Geometry: final body of the model. Coordinates: model frame, mm. Face numbers are marked on the shaded views. A direction names the side the tool comes from. Coordinates: 2 decimals unless noted, no trailing zeros. Order: outer loops, then holes, each group sorted by start corner. A loop starts at its lowest first (then second) coordinate and runs counter-clockwise, first axis right, second up. Notation, with made-up numbers: (-31.75, -26) - (16.25, -26) arc R16 cw to (16.25, -8) - close; hole circle Ø6 at (43, 58). An arc over 180 degrees is marked (long way). Use a Markdown table: item, result. Add a question column.
```python
from build123d import *

# Parameters (mm, degrees)
F1_DEPTH       = 35
F3_D           = 5
F3_START       = 1.7550021
F3_CBORE_D     = 10
F3_CBORE_DEPTH = 8
F4_W           = 22.4
F4_H           = 2
F5_DEPTH       = 25
F6_R           = 6
F7_DEPTH       = 8


with BuildPart() as f1:
    # F0 (on Top) → F1 (new body, symmetric)
    with BuildSketch(Plane.XY):
        with BuildLine():
            ThreePointArc((-17.3192642082, 2.5086026559), (17.5, 0), (-17.3192642082, -2.5086026559))
            Line((-17.3192642082, -2.5086026559), (-20.3459311096, -2.5086026559))
            ThreePointArc((-20.3459311096, -2.5086026559), (-16.3392263155, -12.3806172468), (-7.9192642082, -18.9086026559))
            ThreePointArc((-7.9192642082, -18.9086026559), (20.5, 0), (-7.9192642082, 18.9086026559))
            Line((-7.9192642082, 18.9086026559), (-20.1192642082, 18.9086026559))
            ThreePointArc((-20.1192642082, 18.9086026559), (-25.7761184577, 16.5654569054), (-28.1192642082, 10.9086026559))
            Line((-28.1192642082, 10.9086026559), (-28.1192642082, 2.5086026559))
            Line((-28.1192642082, 2.5086026559), (-17.3192642082, 2.5086026559))
        make_face()
        with BuildLine():
            ThreePointArc((-7.9192642082, -18.9086026559), (-16.3392263155, -12.3806172468), (-20.3459311096, -2.5086026559))
            Line((-20.3459311096, -2.5086026559), (-28.1192642082, -2.5086026559))
            Line((-28.1192642082, -2.5086026559), (-28.1192642082, -10.9086026559))
            ThreePointArc((-28.1192642082, -10.9086026559), (-25.7761184577, -16.5654569054), (-20.1192642082, -18.9086026559))
            Line((-20.1192642082, -18.9086026559), (-7.9192642082, -18.9086026559))
        make_face()
    extrude(amount=F1_DEPTH, both=True)

    # F3 (through all)
    # its depths count from where the whole tool has entered the part; down to there all is cleared
    with Locations(Plane(origin=(0, 18.9086026559, 0), x_dir=(-1, 0, 0), z_dir=(0, 1, 0)).offset(-F3_START)):
        with Locations((20.1192642082, 24.25), (20.1192642082, 9.25), (20.1192642082, -9.25), (20.1192642082, -24.25)):
            CounterBoreHole(F3_D / 2, F3_CBORE_D / 2, F3_CBORE_DEPTH)

    # F4 (on Front) → F5 (cut, symmetric)
    with BuildSketch(Plane.XZ):
        with Locations((-16.9192642082, 0)):
            Rectangle(F4_W, F4_H)
    extrude(amount=F5_DEPTH, both=True, mode=Mode.SUBTRACT)

    # F6 (on face) → F7 (cut)
    with BuildSketch(Plane.XY.offset(35)):
        with Locations((0.8263058844, -25)):
            Circle(F6_R)
        with Locations((18.2619560239, -17.0933830355)):
            Circle(F6_R)
        with Locations((25, 0.8263058844)):
            Circle(F6_R)
        with Locations((17.0933830355, 18.2619560239)):
            Circle(F6_R)
        with Locations((-0.8263058844, 25)):
            Circle(F6_R)
    extrude(amount=-F7_DEPTH, mode=Mode.SUBTRACT)


solid = f1.part
```
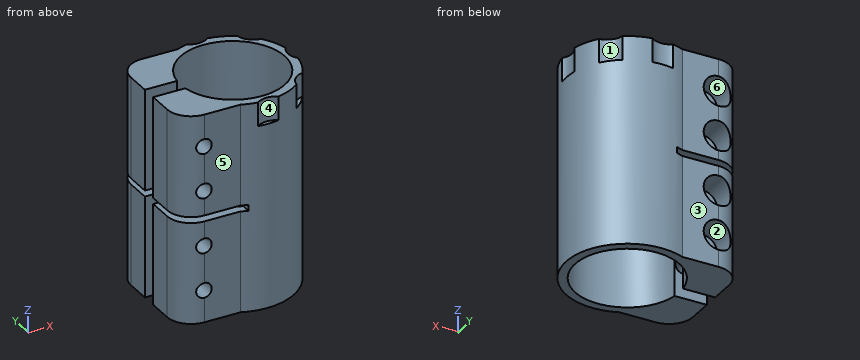
1) Set-up query: the marked faces 4, 5 and 6. Return all of +Z, -Z, +X, -X, +Y, -Y with unobstructed straight access to the full face (end or side cutting, diameter ignored); none if empty.
2) Pin query (flat end, axial travel): pin 1 (0.7 mm diameter, centred on x = -0.5, y = 19.5, fed in from +Z); pin 2 (8 mm diameter, centred on x = -20.12, z = 24.25, fed in from -Y); pin 3 (3.5 mm diameter, centred on x = -11, z = 19, fed in from +Y). Return the tip coordinate at first contact, or that it passes through.
3) Section C-C (z = -24.25). Return loops of the section in (x, y).
4) Draft query along X for the marked faces 1, 2 and 3. Return one class per face: pulls with the +X half, pulls with the -X half, needs draft (parallel to the pull), parting line crosses it, or undercut.
5) Section A-A (y = 10). Return loops of the section in (x, z), then the cut area to 3 significant figures.
6) Section D-D (z = 16.5). Return loops of the section in (x, y).
7) Section B-B (x = 7). Return loops of the section in (y, z).
8) Ray query, line 1 along Z through (x, y) = (-20, -7.5); line 2 along Z through (x, y) = (-21, 16); line 3 along Z through (x, y) = (-13.5, -13). Return the intervals inside material, ascending.
Values follow:
| question | item | result |
|---|---|---|
| 1 | face 4 | +Z, -Y |
| 1 | face 5 | +Z, -Z, -X, -Y |
| 1 | face 6 | +Y |
| 2 | pin 1 | stops at z = 27 |
| 2 | pin 2 | stops at y = -18.91 |
| 2 | pin 3 | stops at y = 18.91 |
| 3 | outline | (-28.12, -10.91) arc R8 ccw to (-22.62, -18.51) - (-22.62, -2.51) - (-28.12, -2.51) - close; (-28.12, 2.51) - (-22.62, 2.51) - (-22.62, 9.15) - (-25.12, 9.15) - (-25.12, 17.15) arc R8 ccw to (-28.12, 10.91) - close; (-17.62, -18.91) - (-7.92, -18.91) arc R20.5 ccw (long way) to (-7.92, 18.91) - (-15.12, 18.91) - (-15.12, 9.15) - (-17.62, 9.15) - (-17.62, 2.51) - (-17.32, 2.51) arc R17.5 cw (long way) to (-17.32, -2.51) - (-17.62, -2.51) - close |
| 4 | face 1 | pulls with the +X half |
| 4 | face 2 | undercut |
| 4 | face 3 | needs draft |
| 5 | outline | (-28.12, -35) - (-14.36, -35) - (-14.36, -1) - (-28.12, -1) - close; (-28.12, 1) - (-14.36, 1) - (-14.36, 35) - (-28.12, 35) - close; (14.36, -35) - (17.9, -35) - (17.9, 35) - (14.36, 35) - close; hole circle Ø10 at (-20.12, -24.25); hole circle Ø10 at (-20.12, -9.25); hole circle Ø10 at (-20.12, 9.25); hole circle Ø10 at (-20.12, 24.25) |
| 5 | area | 869 mm² |
| 6 | outline | (-28.12, -10.91) arc R8 ccw to (-20.12, -18.91) - (-7.92, -18.91) arc R20.5 ccw (long way) to (-7.92, 18.91) - (-20.12, 18.91) arc R8 ccw to (-28.12, 10.91) - (-28.12, 2.51) - (-17.32, 2.51) arc R17.5 cw (long way) to (-17.32, -2.51) - (-28.12, -2.51) - close |
| 7 | outline | (-19.27, -35) - (-16.04, -35) - (-16.04, 35) - (-19.27, 35) - close; (16.04, -35) - (19.27, -35) - (19.27, 35) - (16.04, 35) - close |
| 8 | line 1 | z = -35 to -26.75, -21.75 to -11.75, -6.75 to -1, 1 to 6.75, 11.75 to 21.75, 26.75 to 35 |
| 8 | line 2 | z = -35 to -29.17, -19.33 to -14.17, -4.33 to -1, 1 to 4.33, 14.17 to 19.33, 29.17 to 35 |
| 8 | line 3 | z = -35 to -1, 1 to 35 |
